The model under review builds one solid part; all positions refer to its coordinate system, in mm. Face numbers are marked on the shaded views. Coordinates: 2 decimals unless noted, no trailing zeros. Order: outer loops, then holes, each group sorted by start corner. A loop starts at its lowest first (then second) coordinate and runs counter-clockwise, first axis right, second up. Notation, with made-up numbers: (-31, -32.75) -> (13, -32.75) arc R33 ccw to (13, 4.25) -> close; hole circle Ø10 at (-17, 83.25). An arc over 180 degrees is marked (long way). Answer as CSV lines item,"result". Start each with the question number.
from build123d import *

# Parameters (mm, degrees)
SKETCH1_W           = 40
SKETCH1_H           = 20
SKETCH1_R           = 1.9
BOSS_EXTRUDE1_DEPTH = 4
BOSS_EXTRUDE2_DEPTH = 40
BOSS_EXTRUDE3_START = 20
BOSS_EXTRUDE3_DEPTH = 20
BOSS_EXTRUDE4_DEPTH = 20
FILLET1_R           = 2
BOSS_EXTRUDE5_DEPTH = 2


with BuildPart() as part:
    # Sketch1 → Boss-Extrude1 (new body)
    with BuildSketch(Plane(origin=(0, 0, 0), x_dir=(1, 0, 0), z_dir=(0, 1, 0))):
        with Locations((12.5, 5)):
            Rectangle(SKETCH1_W, SKETCH1_H)
        with Locations(Location((0, 0, 0), (0, 0, 270))):
            Circle(SKETCH1_R, mode=Mode.SUBTRACT)
        with Locations(Location((0, 10, 0), (0, 0, 270))):
            Circle(SKETCH1_R, mode=Mode.SUBTRACT)
        with Locations(Location((25, 10, 0), (0, 0, 90))):
            Circle(SKETCH1_R, mode=Mode.SUBTRACT)
        with Locations(Location((25, 0, 0), (0, 0, 90))):
            Circle(SKETCH1_R, mode=Mode.SUBTRACT)
    extrude(amount=BOSS_EXTRUDE1_DEPTH)

    # Sketch3 → Boss-Extrude2 (add)
    with BuildSketch(Plane(origin=(32.5, 0, 0), x_dir=(0, 0, -1), z_dir=(1, 0, 0))):
        with BuildLine():
            ThreePointArc((22, 0), (20.159285507, 1.837900533), (18.713106366, 4))
            Line((18.713106366, 4), (15, 4))
            Line((15, 4), (15, 0))
            Line((15, 0), (22, 0))
        make_face()
        with BuildLine():
            Line((24.783941732, 20), (21.424248589, 20))
            ThreePointArc((21.424248589, 20), (30.396427812, -3), (39.368607034, 20))
            Line((39.368607034, 20), (36.008913892, 20))
            ThreePointArc((36.008913892, 20), (30.396427812, -1), (24.783941732, 20))
        make_face()
    extrude(amount=-BOSS_EXTRUDE2_DEPTH)

    # Sketch4 → Boss-Extrude3 (add)
    with BuildSketch(Plane(origin=(32.5, 0, 0), x_dir=(0, 0, -1), z_dir=(1, 0, 0)).offset(BOSS_EXTRUDE3_START)):
        with BuildLine():
            Line((24.783941732, 20), (21.424248589, 20))
            ThreePointArc((21.424248589, 20), (30.396427812, -3), (39.368607034, 20))
            Line((39.368607034, 20), (36.008913892, 20))
            ThreePointArc((36.008913892, 20), (30.396427812, -1), (24.783941732, 20))
        make_face()
    extrude(amount=-BOSS_EXTRUDE3_DEPTH)

    # Sketch5 → Boss-Extrude4 (add)
    with BuildSketch(Plane.ZY.offset(7.5)):
        with BuildLine():
            Line((-21.424248589, 20), (-24.783941732, 20))
            ThreePointArc((-24.783941732, 20), (-30.396427812, -1), (-36.008913892, 20))
            Line((-36.008913892, 20), (-39.368607034, 20))
            ThreePointArc((-39.368607034, 20), (-30.396427812, -3), (-21.424248589, 20))
        make_face()
    extrude(amount=BOSS_EXTRUDE4_DEPTH)

    # Fillet1
    fillet1_edges = [part.edges().sort_by_distance(p)[0] for p in [
        (12.5, 4, -18.713106366),
    ]]
    fillet(fillet1_edges, radius=FILLET1_R)

    # Sketch7 → Boss-Extrude5 (add)
    with BuildSketch(Plane.ZY.offset(27.5)):
        with BuildLine():
            Line((-39.368607034, 20), (-21.424248589, 20))
            ThreePointArc((-21.424248589, 20), (-30.396427812, -3), (-39.368607034, 20))
        make_face()
    extrude(amount=BOSS_EXTRUDE5_DEPTH)


solid = part.part
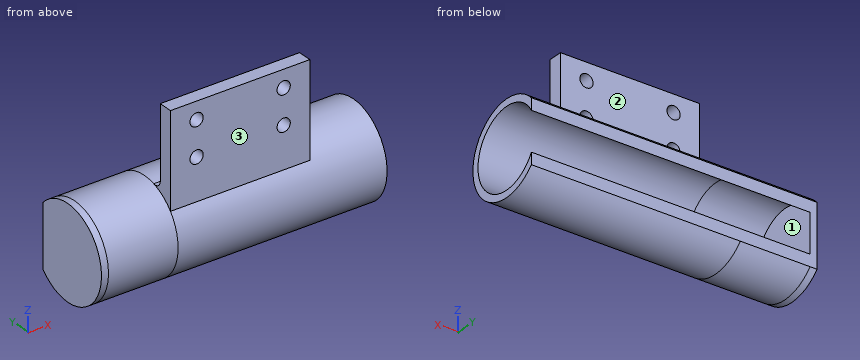
1) Wall thickness on L1, parallel to X at y = 1.25, z = -10; L2, parallel to Z at x = 25, y = 2.45; L3, parallel to Z at x = 25, y = 1.25: over which ranges is each line inside the solid? List them lowest first. Write a range as [from, to].
2) Consider section C-C (y = 10.25). Give the boundary of the cut face in (x, z).
3) Consider section D-D (y = 2). Give the boundary of the cut face in (x, z), plus the area to 3 significant figures.
4) Mouldability with a two-part tool opening along Y and no side actions: class the marked faces 1, 2 and 3 as released by +Y, released by -Y, zero draft, split by the parting line, or undercut.
5) Insertion check: pin 1 Ø3.5 at (x, z) = (0, 0) entering from +Y; pin 2 Ø5 at (y, z) = (3, -13.5) entering from -X; pin 3 Ø6 at (x, z) = (15, -2.5) entering from +Y; pin 4 Ø13.5 at (y, z) = (10.25, -30.4) entering from +X. Each pin has a flat end and moves straight along its axis. Give the tip position at first contact, or say it passes through.
6) Consider section A-A (z = 0). Give the boundary of the cut face in (x, y), plus the area to 3 significant figures.
7) Consider section B-B (x = -1). Give the boundary of the cut face in (y, z), plus the area to 3 significant figures.
Result:
1,L1,"[-7.5, -1.9], [1.9, 23.1], [26.9, 32.5]"
1,L2,"[-41.11, -38.5], [-22.29, -11.9], [-8.1, -1.9], [1.9, 5]"
1,L3,"[-40.12, -37.15], [-23.65, -11.9], [-8.1, -1.9], [1.9, 5]"
2,outline,"(-29.5, -43.65) -> (52.5, -43.65) -> (52.5, -41.65) -> (-27.5, -41.65) -> (-27.5, -19.15) -> (52.5, -19.15) -> (52.5, -17.15) -> (-29.5, -17.15) -> close"
3,outline,"(-29.5, -40.76) -> (52.5, -40.76) -> (52.5, -38.04) -> (-27.5, -38.04) -> (-27.5, -22.75) -> (52.5, -22.75) -> (52.5, -20.03) -> (32.5, -20.03) -> (32.5, 5) -> (-7.5, 5) -> (-7.5, -20.03) -> (-29.5, -20.03) -> close; hole circle Ø3.8 at (0, -10); hole circle Ø3.8 at (0, 0); hole circle Ø3.8 at (25, -10); hole circle Ø3.8 at (25, 0)"
3,area,"1,430 mm2"
4,face 1,"undercut"
4,face 2,"released by +Y"
4,face 3,"released by -Y"
5,pin 1,"through"
5,pin 2,"x = -7.5"
5,pin 3,"y = 4"
5,pin 4,"x = -27.5"
6,outline,"(-7.5, 0) -> (-1.9, 0) -> (-1.9, 4) -> (-7.5, 4) -> close; (1.9, 0) -> (23.1, 0) -> (23.1, 4) -> (1.9, 4) -> close; (26.9, 0) -> (32.5, 0) -> (32.5, 4) -> (26.9, 4) -> close"
6,area,"130 mm2"
7,outline,"(0, -22) arc R13.25 ccw to (20, -39.37) -> (20, -36.01) arc R11.25 cw (long way) to (20, -24.78) -> (20, -21.42) arc R13.25 ccw to (6.56, -17.67) arc R2 cw to (4, -15.75) -> (4, -11.62) -> (0, -11.62) -> close; (0, -8.38) -> (4, -8.38) -> (4, -1.62) -> (0, -1.62) -> close; (0, 1.62) -> (4, 1.62) -> (4, 5) -> (0, 5) -> close"
7,area,"199 mm2"
